from build123d import *

# Parameters (mm, degrees)
F0_R     = 15.875
F1_DEPTH = 8.89
F4_W     = 2.032
F4_H     = 3.302
F5_ANGLE = -60


with BuildPart() as f1:
    # F0 (on Top) → F1 (new body)
    with BuildSketch(Plane.XY):
        Circle(F0_R)
    extrude(amount=F1_DEPTH)

    # F2 (on Front) → F3 (revolve, cut)
    with BuildSketch(Plane.XZ):
        Polygon((11.43, 6.35), (0, 6.35), (0, 0), (9.398, 0), (9.398, 3.302), (11.43, 3.302), align=None)
    revolve(axis=Axis((0, 0, 3.175), (0, 0, 1)), mode=Mode.SUBTRACT)

    # F4 (on Front) → F5 (revolve, cut)
    with BuildSketch(Plane.XZ):
        with Locations((10.414, 1.651)):
            Rectangle(F4_W, F4_H)
    revolve(axis=Axis((0, 0, 3.175), (0, 0, 1)), revolution_arc=F5_ANGLE, mode=Mode.SUBTRACT)


solid = f1.part
Build history of the part. All positions in model axes, mm. A direction names the side the tool comes from. Round coordinates to 2 decimals unless told otherwise and drop trailing zeros. Loops run counter-clockwise (first coordinate to the right, second up) from the corner with the lowest first, then second, coordinate; pieces in that order, holes last. Notation, with made-up numbers: (81, -25) -> (89, -25) arc R29 cw to (89, 5) -> close; hole circle Ø8 at (30.5, 19). An arc over 180 degrees is marked (long way). Answer in a Markdown table with one row per item.
Item 1: Saw through at B-B (y = -2). Write the cut outline in (x, z), and give its area (3 significant figures).
Answers below:
| item | result |
|---|---|
| outline | (-15.75, 0) -> (-9.18, 0) -> (-9.18, 3.3) -> (-11.25, 3.3) -> (-11.25, 6.35) -> (11.25, 6.35) -> (11.25, 0) -> (15.75, 0) -> (15.75, 8.89) -> (-15.75, 8.89) -> close |
| area | 144 mm² |
Item 2: Saw through at C-C (z = 4). Write the cut outline in (x, y) (3 decimals).
Answers below:
| item | result |
|---|---|
| outline | circle Ø31.75 at (0, 0); hole circle Ø22.86 at (0, 0) |
Item 3: Pin check, flat tips, straight feed: pin 1 (0.6 mm diameter, centred on x = 10, z = 1.5, fed in from -Y); pin 2 (1.5 mm diameter, centred on y = -5, z = 8, fed in from +X); pin 3 (3 mm diameter, centred on y = 2, z = 4, fed in from +X). Stop position of each tip, or through.
Answers below:
| item | result |
|---|---|
| pin 1 | stops at y = -12.57 |
| pin 2 | stops at x = 15.3 |
| pin 3 | stops at x = 15.87 |
Item 4: Drill centre lines: L1, parallel to Y at x = 0, z = 4.7 (3 decimals); L2, parallel to Z at x = -2.5, y = 10; L3, parallel to Y at x = 0, z = 0.95 (3 decimals). Where is each one in solid material? Low to high. Write a range as [from, to].
Answers below:
| item | result |
|---|---|
| L1 | y = [-15.875, -11.43], [11.43, 15.875] |
| L2 | z = [0, 3.3], [6.35, 8.89] |
| L3 | y = [-15.875, -9.398], [9.398, 15.875] |
Item 5: Saw through at A-A (x = 0). Write the cut outline in (y, z) (3 decimals), and give its area (3 significant figures).
Answers below:
| item | result |
|---|---|
| outline | (-15.875, 0) -> (-9.398, 0) -> (-9.398, 3.302) -> (-11.43, 3.302) -> (-11.43, 6.35) -> (11.43, 6.35) -> (11.43, 3.302) -> (9.398, 3.302) -> (9.398, 0) -> (15.875, 0) -> (15.875, 8.89) -> (-15.875, 8.89) -> close |
| area | 151 mm² |
Item 6: Saw through at D-D (x = 8.5). Write the cut outline in (y, z), and give its area (3 significant figures).
Answers below:
| item | result |
|---|---|
| outline | (-13.41, 0) -> (-7.64, 0) -> (-7.64, 6.35) -> (7.64, 6.35) -> (7.64, 3.3) -> (4.01, 3.3) -> (4.01, 0) -> (13.41, 0) -> (13.41, 8.89) -> (-13.41, 8.89) -> close |
| area | 153 mm² |
Item 7: Mould opens along Z. For faces 4 (the flat face through (5.2, -9.01, 1.67)), 5 (the flat face through (0, 0, 6.35)), 6 (the flat face through (-7, -7, 0)), 7 (the flat face through (0, 0, 8.89)) say: +Z half, -Z half, draft (parallel to the pull), parting line (faces both ways), or undercut.
Answers below:
| item | result |
|---|---|
| face 4 | draft |
| face 5 | undercut |
| face 6 | -Z half |
| face 7 | +Z half |
Item 8: Which spindle directions (+Z, -Z, +X, -X, +Y, -Y) get a long thin tool onto all of the face, cutting with end or side? Do faces 1 (the cylindrical face through (-3.441, -15.497, 4.383)), 2 (the flat face through (-6, 8, 3.302)), 3 (the cylindrical face through (-7.961, 4.994, 1.674)). Say none if no direction does.
Answers below:
| item | result |
|---|---|
| face 1 | +Z, -Z |
| face 2 | none |
| face 3 | -Z |
